Verification items for the finished model (mm, model axes). Face numbers are marked on the shaded views. A direction names the side the tool comes from. Coordinates: 2 decimals unless noted, no trailing zeros. Write each loop counter-clockwise with the first axis right and the second up, starting at its lowest first coordinate (ties: lowest second). Pieces come first, ordered by that corner, then holes. Notation, with made-up numbers: M 79,50 L 132,50 A22 cw 132,68 Z; hole C 22,-3.5 d4. An arc over 180 degrees is marked long. Answer in a Markdown table with one row per item.
from build123d import *

# Parameters (mm, degrees)
F1_DEPTH = 179.578
F2_F1_R  = 15.3302561211
F2_F2_R  = 15.3302561211


with BuildPart() as f1:
    # F0 (on Front) → F1 (new body)
    with BuildSketch(Plane.XZ):
        with BuildLine():
            Line((-60.1250007749, 41.0845763981), (-99.0082323551, 41.0845763981))
            Line((-99.0082323551, 41.0845763981), (-99.0082323551, -33.9665971696))
            Line((-99.0082323551, -33.9665971696), (36.3630242646, -33.9665971696))
            Line((36.3630242646, -33.9665971696), (36.3630242646, 41.0845763981))
            Line((36.3630242646, 41.0845763981), (-15.4812876135, 41.0845763981))
            Line((-15.4812876135, 41.0845763981), (-15.4812876135, 66.3503706455))
            ThreePointArc((-15.4812876135, 66.3503706455), (-37.8031441942, 124.2664472866), (-60.1250007749, 66.3503706455))
            Line((-60.1250007749, 66.3503706455), (-60.1250007749, 41.0845763981))
        make_face()
    extrude(amount=F1_DEPTH)

    # F2: fillet of radius 15.3302561211 on 14 edges, made by hand

    # F2_f1
    f2_f1_edges = [f1.edges().sort_by_distance(p)[0] for p in [
        (-15.4812876135, -89.789, 41.0845763981),
    ]]
    fillet(f2_f1_edges, radius=F2_F1_R)

    # F2_f2
    f2_f2_edges = [f1.edges().sort_by_distance(p)[0] for p in [
        (36.3630242646, -89.789, 41.0845763981),
        (18.1059963861, 0, 41.0845763981),
        (18.1059963861, -179.578, 41.0845763981),
        (-99.0082323551, -89.789, -33.9665971696),
        (36.3630242646, -89.789, -33.9665971696),
        (-31.3226040453, 0, -33.9665971696),
        (-31.3226040453, -179.578, -33.9665971696),
        (-37.8031441942, -179.578, 124.2664472866),
        (-60.1250007749, -179.578, 53.7174735218),
        (-79.566616565, -179.578, 41.0845763981),
        (-99.0082323551, -179.578, 3.5589896142),
        (36.3630242646, -179.578, 3.5589896142),
        (-15.4812876135, -179.578, 61.3826015824),
        (-10.991159553, -179.578, 45.5747044587),
        (-10.991159553, 0, 45.5747044587),
    ]]
    fillet(f2_f2_edges, radius=F2_F2_R)


solid = f1.part
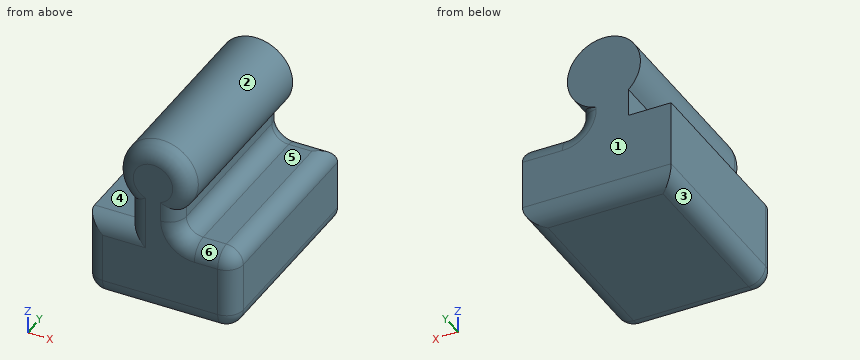
1) Tool access check on the marked faces 4, 5 and 6. Record the directions out of +Z, -Z, +X, -X, +Y, -Y that give a thin tool (end or side, any length) a straight path to the whole face; none if there is none.
Response values:
| item | result |
|---|---|
| face 4 | -X, +Y, -Y |
| face 5 | +Z, +X, +Y, -Y |
| face 6 | +Z, +X, -Y |
2) Sectioned sample at B-B (x = -73.5). Record the cut outline in (y, z).
Response values:
| item | result |
|---|---|
| outline | M -179.58,-18.64 A15.33 ccw -164.25,-33.97 L -15.33,-33.97 A15.33 ccw 0,-18.64 L 0,41.08 L -164.25,41.08 A15.33 ccw -179.58,25.75 Z |
3) Release check for a two-part mould opening along Z. For the marked faces 1, 2 and 3 record: +Z half, -Z half, draft (parallel to the pull), parting line (faces both ways), or undercut.
Response values:
| item | result |
|---|---|
| face 1 | draft |
| face 2 | undercut |
| face 3 | -Z half |
4) Depth check by flat-ended pin: pin 1 (6.5 mm diameter, centred on x = 11, y = -102, fed in from +Z); pin 2 (12 mm diameter, centred on x = -75, z = 32, fed in from -Y); pin 3 (1.5 mm diameter, centred on y = -102.5, z = 61, fed in from +X). Enter the tip coordinate at first touch or a pass-through.
Response values:
| item | result |
|---|---|
| pin 1 | stops at z = 41.08 |
| pin 2 | stops at y = -179.58 |
| pin 3 | stops at x = -15.48 |
5) Sectioned sample at A-A (y = -36). Record the cut outline in (x, z) (3 decimals).
Response values:
| item | result |
|---|---|
| outline | M -99.008,-18.636 A15.33 ccw -83.678,-33.967 L 21.033,-33.967 A15.33 ccw 36.363,-18.636 L 36.363,25.754 A15.33 ccw 21.033,41.085 L -0.151,41.085 A15.33 cw -15.481,56.415 L -15.481,66.35 A33.26 ccw long -60.125,66.35 L -60.125,41.085 L -99.008,41.085 Z |
6) Sectioned sample at C-C (z = 63). Record the cut outline in (x, y) (3 decimals), then the cut area to 3 significant figures.
Response values:
| item | result |
|---|---|
| outline | M -60.125,-164.248 A15.33 ccw -44.795,-179.578 L -30.812,-179.578 A15.33 ccw -15.481,-164.248 L -15.481,-15.33 A15.33 ccw -19.864,-4.599 L -19.864,0 L -60.125,0 Z |
| area | 7,880 mm² |
7) Thickness scan on L1, parallel to Y at x = -46, z = 64; L2, parallel to Z at x = 15, y = -51.5; L3, parallel to Z at x = 22, y = -160. Record the ranges inside material, lowest first. Write a range as [from, to].
Response values:
| item | result |
|---|---|
| L1 | y = [-179.53, 0] |
| L2 | z = [-33.97, 41.08] |
| L3 | z = [-33.94, 41.05] |
